For this review, use the dimensioned drawing (mm, ordinates from the lowest corner) and the shaded views. A direction names the side the tool comes from. Coordinates: 2 decimals unless noted, no trailing zeros. Order: outer loops, then holes, each group sorted by start corner. A loop starts at its lowest first (then second) coordinate and runs counter-clockwise, first axis right, second up. Notation, with made-up numbers: M 75,-26 L 94,-26 A28 cw 94,12 Z; hole C 70.5,84.25 d8. An arc over 180 degrees is marked long. Answer in a Markdown table with one row per item.
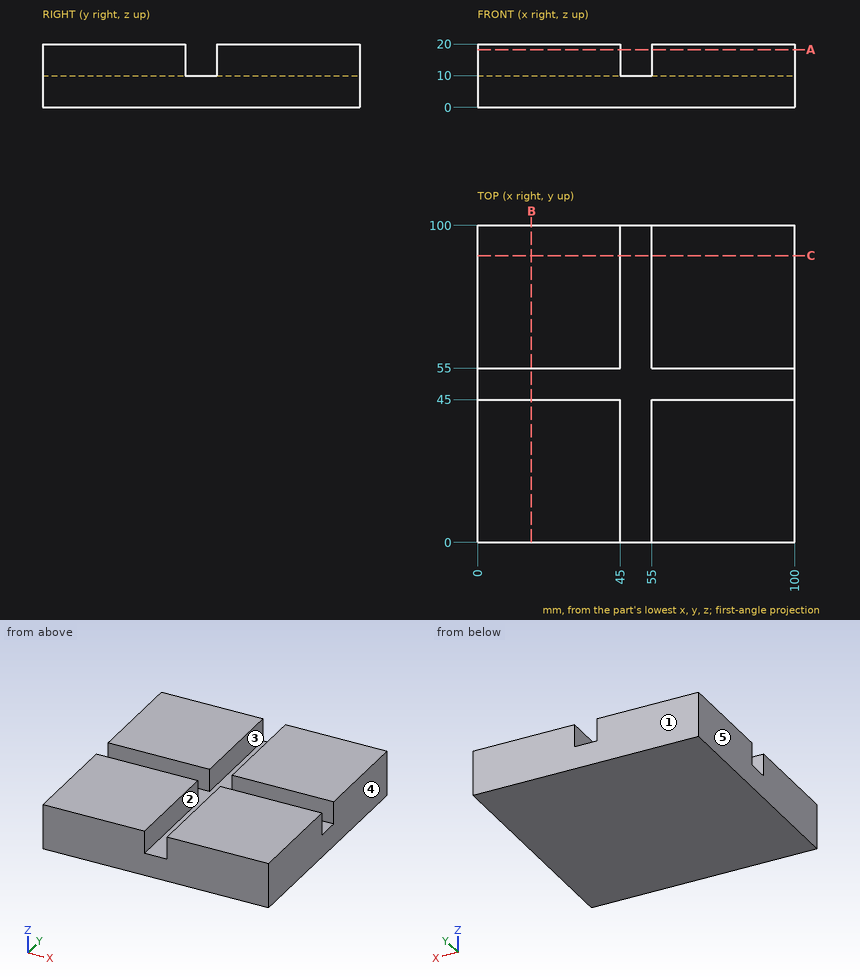
(1) For the marked faces 1 and 2, list the 3-axis set-ups (+Z, -Z, +X, -X, +Y, -Y) from which the entire face can be reached by the end or side of a thin tool; tool diameter is ignored.
Return value:
| item | result |
|---|---|
| face 1 | +Z, -Z, +X, -X, +Y |
| face 2 | +Z, +Y, -Y |
(2) Add section B-B, the plane x = 17. Give the boundary of the cut face in (y, z), and give its area (3 significant figures).
Return value:
| item | result |
|---|---|
| outline | M 0,0 L 100,0 L 100,20 L 55,20 L 55,10 L 45,10 L 45,20 L 0,20 Z |
| area | 1,900 mm2 |
(3) Insertion check: pin 1 Ø1 at (x, y) = (50, 83.5) entering from +Z. The pin has a flat end and moves straight along its axis. Give the tip position at first contact, or say it passes through.
Return value:
| item | result |
|---|---|
| pin 1 | stops at z = 10 |
(4) For line 1 along X through (y, z) = (79, 13); line 2 along Z through (x, y) = (49, 96), list the stretches that pass through material, from the lowest coordinate up. Write a range as from..to.
Return value:
| item | result |
|---|---|
| line 1 | x = 0..45, 55..100 |
| line 2 | z = 0..10 |
(5) Add section A-A, the plane z = 18.25. Give the boundary of the cut face in (x, y), and give its area (3 significant figures).
Return value:
| item | result |
|---|---|
| outline | M 0,0 L 45,0 L 45,45 L 0,45 Z; M 0,55 L 45,55 L 45,100 L 0,100 Z; M 55,0 L 100,0 L 100,45 L 55,45 Z; M 55,55 L 100,55 L 100,100 L 55,100 Z |
| area | 8,100 mm2 |
(6) Draft analysis for pull direction X (two halves, no side actions). For the marked faces 3, 4 and 5, state which applies: pulls with the +X half, pulls with the -X half, needs draft (parallel to the pull), parting line crosses it, or undercut.
Return value:
| item | result |
|---|---|
| face 3 | undercut |
| face 4 | pulls with the +X half |
| face 5 | pulls with the -X half |
